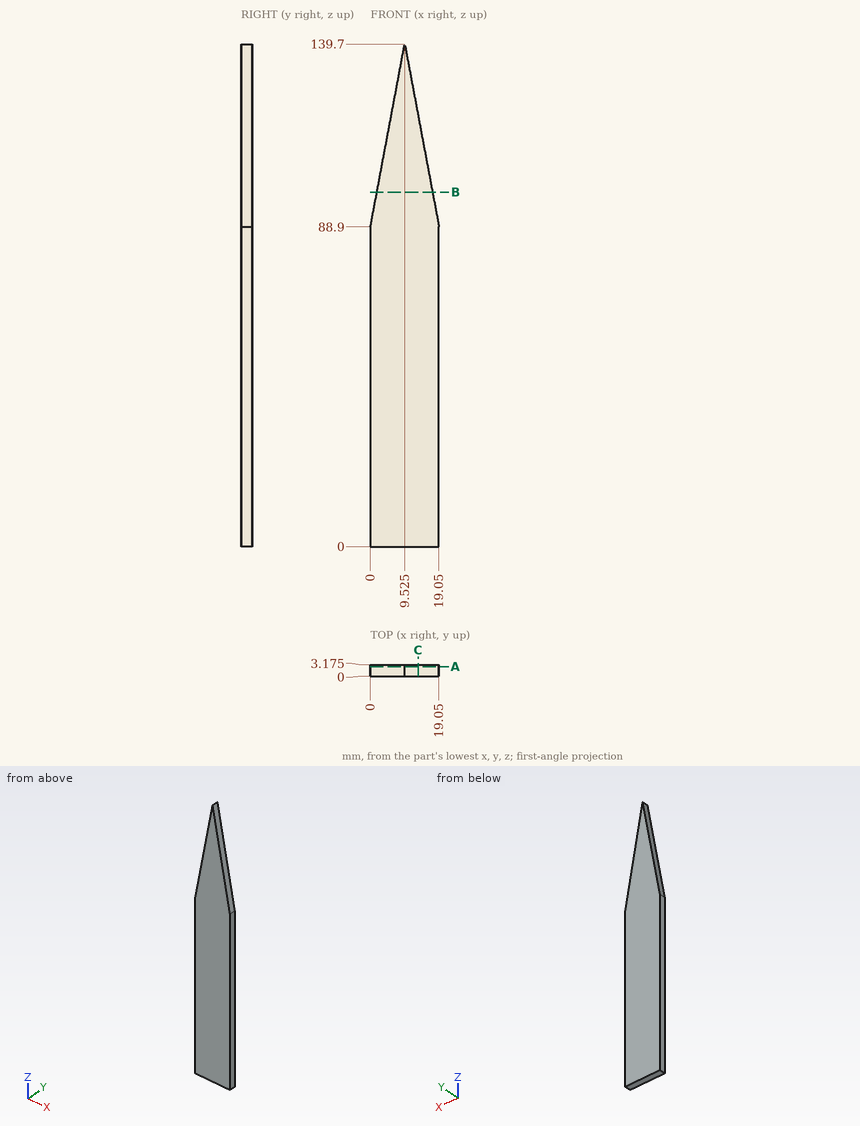
Answer from the drawing. Dimensions are ordinates in mm from the lowest x, y and z of the part. Give positions to 0.01 mm unless a question says otherwise; leave off trailing zeros. Write each loop counter-clockwise with the first axis right and the second up, starting at its lowest first coordinate (ties: lowest second). Pieces come first, ordered by that corner, then holes. Notation, with made-up numbers: (-0.5, -9.75) -> (7.5, -9.75) arc R36 cw to (7.5, 29.25) -> close; hole circle Ø2 at (35, 24). An arc over 180 degrees is marked (long way). Use a Markdown table: item, result.
(1) Find the intervals of material crossed by probe 1 along X at (y, z) = (1.3, 91.5); probe 2 along X at (y, z) = (1.1, 115), in increasing order. Write a range as from..to.
Return value:
| item | result |
|---|---|
| probe 1 | 0.49..18.56 |
| probe 2 | 4.89..14.16 |
(2) Section A-A, the plane y = 2.6 is taken. Determine the outline of the cut face in (x, z) (3 decimals), then the cut area to 3 significant figures.
Return value:
| item | result |
|---|---|
| outline | (0, 0) -> (19.05, 0) -> (19.05, 88.9) -> (9.525, 139.7) -> (0, 88.9) -> close |
| area | 2,180 mm2 |
(3) Section B-B, the plane z = 98.5 is taken. Determine the outline of the cut face in (x, y) (3 decimals), then the cut area to 3 significant figures.
Return value:
| item | result |
|---|---|
| outline | (1.8, 0) -> (17.25, 0) -> (17.25, 3.175) -> (1.8, 3.175) -> close |
| area | 49.1 mm2 |
(4) Section C-C, the plane x = 13.25 is taken. Determine the outline of the cut face in (y, z) (3 decimals), then the cut area to 3 significant figures.
Return value:
| item | result |
|---|---|
| outline | (0, 0) -> (3.175, 0) -> (3.175, 119.833) -> (0, 119.833) -> close |
| area | 380 mm2 |
